CAD build for the part. Positions are in the model's coordinates, mm. Face numbers are marked on the shaded views. A direction names the side the tool comes from. Round coordinates to 2 decimals unless told otherwise and drop trailing zeros. Loops run counter-clockwise (first coordinate to the right, second up) from the corner with the lowest first, then second, coordinate; pieces in that order, holes last. Notation, with made-up numbers: (53, -16.75) -> (78, -16.75) arc R35 cw to (78, 19.25) -> close; hole circle Ø5 at (51, 25). An arc over 180 degrees is marked (long way). Answer as CSV lines item,"result".
```python
from build123d import *

# Parameters (mm, degrees)
BOSS_EXTRUDE1_DEPTH      = 7
BOSS_EXTRUDE1_DEPTH_BACK = 7
CUT_EXTRUDE1_DEPTH       = 15
SKETCH3_R                = 2.5
CUT_EXTRUDE2_DEPTH       = 7.5


with BuildPart() as part:
    # Sketch1 → Boss-Extrude1 (new body, two sides)
    with BuildSketch(Plane.XY) as boss_extrude1_sk:
        Polygon((9, 3.25), (21, 3.25), (21, -3.25), (-21, -3.25), (-21, 3.25), (-9, 3.25), (-9, 29.75), (9, 29.75), align=None)
    extrude(amount=BOSS_EXTRUDE1_DEPTH)
    extrude(boss_extrude1_sk.sketch, amount=-BOSS_EXTRUDE1_DEPTH_BACK)

    # Sketch2 → Cut-Extrude1 (cut, through all)
    with BuildSketch(Plane.XY.offset(7)):
        with BuildLine():
            Line((-0.5, 20.718626967), (-0.5, 29.75))
            Line((-0.5, 29.75), (0.5, 29.75))
            Line((0.5, 29.75), (0.5, 20.718626967))
            ThreePointArc((0.5, 20.718626967), (0, 12.75), (-0.5, 20.718626967))
        make_face()
    extrude(amount=-CUT_EXTRUDE1_DEPTH, mode=Mode.SUBTRACT)

    # Sketch3 → Cut-Extrude2 (cut, through all)
    with BuildSketch(Plane(origin=(0, 3.25, 0), x_dir=(1, 0, 0), z_dir=(0, 1, 0))):
        with Locations((16, 0)):
            Circle(SKETCH3_R)
        with Locations((-16, 0)):
            Circle(SKETCH3_R)
    extrude(amount=-CUT_EXTRUDE2_DEPTH, mode=Mode.SUBTRACT)


solid = part.part
```
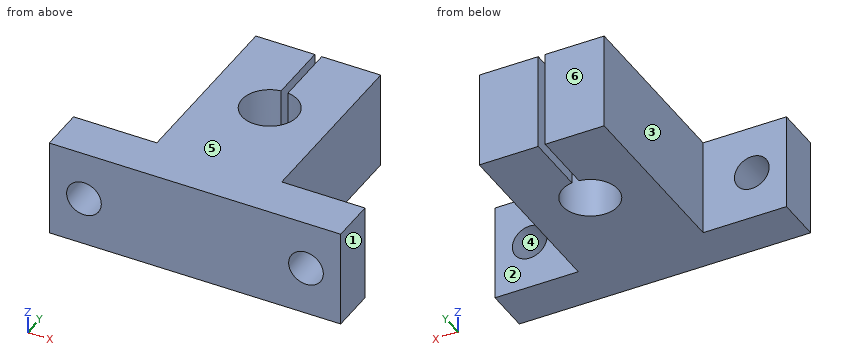
Q1. Slice it at A-A, the plane z = 0. Give the cut face in (x, y), and give its area (3 significant figures).
Results:
outline,"(-21, -3.25) -> (-18.5, -3.25) -> (-18.5, 3.25) -> (-21, 3.25) -> close; (-13.5, -3.25) -> (13.5, -3.25) -> (13.5, 3.25) -> (9, 3.25) -> (9, 29.75) -> (0.5, 29.75) -> (0.5, 20.72) arc R4 cw (long way) to (-0.5, 20.72) -> (-0.5, 29.75) -> (-9, 29.75) -> (-9, 3.25) -> (-13.5, 3.25) -> close; (18.5, -3.25) -> (21, -3.25) -> (21, 3.25) -> (18.5, 3.25) -> close"
area,"626 mm2"
Q2. Slice it at C-C, the plane y = 16.75. Give the cut face in (x, z).
Results:
outline,"(-9, -7) -> (-4, -7) -> (-4, 7) -> (-9, 7) -> close; (4, -7) -> (9, -7) -> (9, 7) -> (4, 7) -> close"
Q3. Slice it at B-B, the plane x = 16. Give the cut face in (y, z).
Results:
outline,"(-3.25, -7) -> (3.25, -7) -> (3.25, -2.5) -> (-3.25, -2.5) -> close; (-3.25, 2.5) -> (3.25, 2.5) -> (3.25, 7) -> (-3.25, 7) -> close"
Q4. Probe L1, parallel to X at y = -0.25, z = 0; L2, parallel to X at y = 28.5, z = -1.5; L3, parallel to Y at x = 2.5, z = 6. List the from-to ranges inside material, lowest first. Write a range as [from, to].
Results:
L1,"[-21, -18.5], [-13.5, 13.5], [18.5, 21]"
L2,"[-9, -0.5], [0.5, 9]"
L3,"[-3.25, 13.63], [19.87, 29.75]"
Q5. Drop flat-ended pins along their axis: pin 1 Ø1 at (y, z) = (22.5, -4.5) entering from -X; pin 2 Ø4 at (y, z) = (23, 1.5) entering from +X; pin 3 Ø4.5 at (x, z) = (16, 0) entering from -Y; pin 4 Ø3.5 at (x, z) = (-15.5, 1) entering from +Y. Give the stop position or say it passes through.
Results:
pin 1,"x = -9"
pin 2,"x = 9"
pin 3,"through"
pin 4,"y = 3.25"
Q6. Slice it at D-D, the plane z = -5.25. Give the cut face in (x, y).
Results:
outline,"(-21, -3.25) -> (21, -3.25) -> (21, 3.25) -> (9, 3.25) -> (9, 29.75) -> (0.5, 29.75) -> (0.5, 20.72) arc R4 cw (long way) to (-0.5, 20.72) -> (-0.5, 29.75) -> (-9, 29.75) -> (-9, 3.25) -> (-21, 3.25) -> close"
Q7. Two-plate mould, pull along Z, no slides. Class the marked faces 4, 5 and 6: pulls with the +Z half, pulls with the -Z half, needs draft (parallel to the pull), parting line crosses it, or undercut.
Results:
face 4,"undercut"
face 5,"pulls with the +Z half"
face 6,"needs draft"
Q8. Tool access for the marked faces 1, 2 and 3: list every direction of +Z, -Z, +X, -X, +Y, -Y with a clear straight run to the whole face (end or side of a thin tool).
Results:
face 1,"+Z, -Z, +X, +Y, -Y"
face 2,"+Z, -Z, +X, +Y"
face 3,"+Z, -Z, -X, +Y"
